```python
from build123d import *

# Parameters (mm, degrees)
F1_DEPTH = 62.5
F0_W     = 21.2285545291
F0_H     = 18
F2_DEPTH = 25


with BuildPart() as f1:
    # F0 (on Front) → F1 (new body, symmetric)
    with BuildSketch(Plane.XZ):
        Polygon((-41, 10), (-41, -10), (41, -10), (41, 10), (23, 10), align=None)
    extrude(amount=F1_DEPTH, both=True)

    # F0 (on Front) → F2 (join, symmetric)
    with BuildSketch(Plane.XZ):
        with BuildLine():
            Line((23, 10), (41, 10))
            Line((41, 10), (41, 25))
            ThreePointArc((41, 25), (45.686291501, 36.313708499), (57, 41))
            Line((57, 41), (60, 41))
            Line((60, 41), (60, 59))
            Line((60, 59), (57, 59))
            add(Edge.make_bspline(
                [(55.3022101566, 58.9575839784), (55.8715194046, 58.9754471326), (56.4375192282, 58.9895954178), (57, 59)],
                knots=[108.0329717794, 108.0329717794, 108.0329717794, 108.0329717794, 109.5673308975, 109.5673308975, 109.5673308975, 109.5673308975], degree=3))
            ThreePointArc((55.3022101566, 58.9575839784), (32.3654221198, 48.4336845729), (23, 25))
            Line((23, 25), (23, 10))
        make_face()
        with Locations((70.6142772645, 50)):
            Rectangle(F0_W, F0_H)
        Polygon((60, 65), (60, 59), (81.2285545291, 59), (81.2285545291, 41), (60, 41), (60, 37), (110, 37), (110, 65), align=None)
    extrude(amount=F2_DEPTH, both=True)


solid = f1.part
```
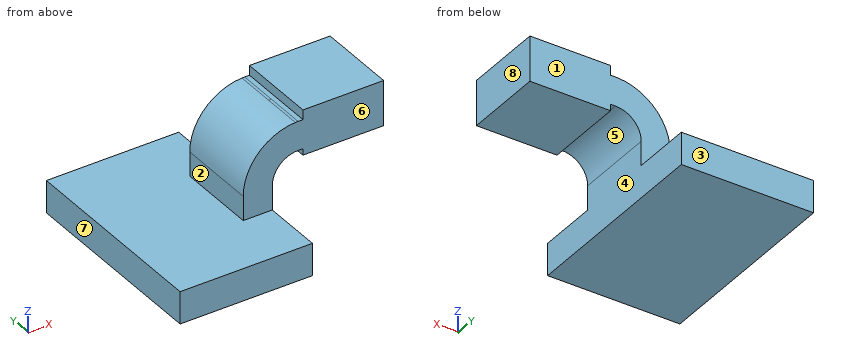
Can you work these out from the model? Positions are in its coordinate system, mm. Face numbers are marked on the shaded views. A direction names the side the tool comes from. Coordinates: 2 decimals unless noted, no trailing zeros. Loops run counter-clockwise (first coordinate to the right, second up) from the corner with the lowest first, then second, coordinate; pieces in that order, holes last.
1) For pin 1 (1 mm diameter, centred on y = 19.5, z = 11.5, fed in from -X); pin 2 (24.5 mm diameter, centred on x = -9.5, y = -1.5, fed in from +Z); pin 3 (2 mm diameter, centred on y = 12, z = 39, fed in from -X), each with a flat end and sliding along its axis, tell me the tip position at first contact or that it passes through.
2) Imagine slicing it at B-B on y = -42.5. List the corners of the cut face in (x, z) for me.
3) Thinking about a two-plate mould opening in X: for the marked faces 5, 6, 7 and 8, which applies, pulls with the +X half, pulls with the -X half, needs draft (parallel to the pull), parting line crosses it, or undercut?
4) I need wall thicknesses on probe 1 along X at (y, z) = (20, -5.5); probe 2 along Y at (x, z) = (67.5, 61); probe 3 along X at (y, z) = (-22, 14.5). Which ranges of each line are inside material? Lowest first, please.
5) Which directions (+Z, -Z, +X, -X, +Y, -Y) give clear straight access to the entire face, cutting with the end or side of a thin tool? Please do the marked faces 1, 2, 3 and 4.
6) Imagine slicing it at A-A on z = 15. List the corners of the cut face in (x, y) for me, plus the area to 3 significant figures.
Completed:
1. pin 1: stops at x = 23
1. pin 2: stops at z = 10
1. pin 3: stops at x = 25.58
2. outline: (-41, -10) - (41, -10) - (41, 10) - (-41, 10) - close
3. face 5: undercut
3. face 6: needs draft
3. face 7: pulls with the -X half
3. face 8: pulls with the +X half
4. probe 1: x = -41 to 41
4. probe 2: y = -25 to 25
4. probe 3: x = 23 to 41
5. face 1: +Z, +X, -X, +Y
5. face 2: +Z, -X, +Y, -Y
5. face 3: +Z, -Z, +X, -X, +Y
5. face 4: -Z, +X, +Y, -Y
6. outline: (23, -25) - (41, -25) - (41, 25) - (23, 25) - close
6. area: 900 mm2
